Source: CAD feature listing. Evaluate the final solid. Frame: model axes, mm. A direction names the side the tool comes from. Give positions to 0.01 mm unless a question says otherwise; leave off trailing zeros. Order: outer loops, then holes, each group sorted by start corner. A loop starts at its lowest first (then second) coordinate and runs counter-clockwise, first axis right, second up. Notation, with made-up numbers: M 66,83 L 123,83 A27 ccw 123,122 Z; hole C 0,13.25 d3. An arc over 180 degrees is marked long. Use CSV: the item, a comma, the result in double quotes. Start each with the question number.
Item 1: Section query D-D on z = 16.5. Return loops of the section in (x, y), and give its area (3 significant figures).
Item 2: Section query B-B on z = 56. Return loops of the section in (x, y), and give its area (3 significant figures).
Item 3: Pull-direction query (Z, two-part tool) for faces 5 (the face through (3.1, 5.3, 45.72)), 6 (the face through (4.041, 3, 54)), 7 (the face through (0, 0, 0)), 8 (the face through (-1.26, -5.674, 26.146)); classes: +Z half, -Z half, draft (parallel to the pull), parting line (faces both ways), or undercut.
Item 4: Section query C-C on x = -5. Return loops of the section in (y, z).
Item 5: Access query for faces 1 (the face through (-3.639, 3, 54)), 2 (the face through (0, 5.812, 54)), 3 (the face through (-2.8, 5.4, 45.72)), 4 (the face through (0, 0.732, 54)). Directions: +Z, -Z, +X, -X, +Y, -Y. A direction counts if a zero-diameter tool reaches every point of the face in a straight line with its end or side. Return the directions, or none.
Item 6: First-contact query: pin 1 (10 mm diameter, centred on y = 7.5, z = 24.5, fed in from +X); pin 2 (8 mm diameter, centred on x = -8.5, z = 40.5, fed in from -Y); pin 3 (8.5 mm diameter, centred on x = -1, z = 57, fed in from +Y). Flat tips, straight axial feed; report the tip coordinate or a pass-through.
Item 7: Ray query, probe 1 along Z at (x, y) = (-2.5, 5.75); probe 2 along Z at (x, y) = (7.25, 2.25); probe 3 along X at (y, z) = (1.5, 51.5). Return the intervals inside material, ascending. Write a range as from..to.
Item 8: Section query A-A on y = 0. Return loops of the section in (x, z).
from build123d import *

# Parameters (mm, degrees)
F0_R     = 12.7
F1_DEPTH = 7.112
F2_R     = 5.811931
F3_DEPTH = 38.608
F5_DEPTH = 17.526


with BuildPart() as f1:
    # F0 (on Top) → F1 (new body)
    with BuildSketch(Plane.XY):
        Circle(F0_R)
    extrude(amount=F1_DEPTH)

    # F2 (on face) → F3 (join)
    with BuildSketch(Plane.XY.offset(7.112)):
        Circle(F2_R)
    extrude(amount=F3_DEPTH)

    # F4 (on face) → F5 (join)
    with BuildSketch(Plane.XY.offset(45.72)):
        with BuildLine():
            ThreePointArc((4.041356, 4.176839), (2.179798, 5.387673), (0, 5.811931))
            ThreePointArc((0, 5.811931), (-1.928979, 5.482479), (-3.639269, 4.531475))
            Line((-3.639269, 4.531475), (-3.639269, 0.731931))
            Line((-3.639269, 0.731931), (4.041356, 0.731931))
            Line((4.041356, 0.731931), (4.041356, 4.176839))
        make_face()
        with BuildLine():
            ThreePointArc((-3.639269, 4.531475), (-1.928979, 5.482479), (0, 5.811931))
            Line((0, 5.811931), (-3.639269, 5.811931))
            Line((-3.639269, 5.811931), (-3.639269, 4.531475))
        make_face()
        with BuildLine():
            Line((4.041356, 4.176839), (4.041356, 5.811931))
            Line((4.041356, 5.811931), (0, 5.811931))
            ThreePointArc((0, 5.811931), (2.179798, 5.387673), (4.041356, 4.176839))
        make_face()
    extrude(amount=F5_DEPTH)


solid = f1.part
Verdict:
1,outline,"C 0,0 d11.62"
1,area,"106 mm2"
2,outline,"M -3.64,0.73 L 4.04,0.73 L 4.04,5.81 L -3.64,5.81 Z"
2,area,"39.0 mm2"
3,face 5,"undercut"
3,face 6,"draft"
3,face 7,"-Z half"
3,face 8,"undercut"
4,outline,"M -11.67,0 L 11.67,0 L 11.67,7.11 L 2.96,7.11 L 2.96,45.72 L -2.96,45.72 L -2.96,7.11 L -11.67,7.11 Z"
5,face 1,"+Z, -X, +Y, -Y"
5,face 2,"+Z, +X, -X, +Y"
5,face 3,"-X, +Y"
5,face 4,"+Z, +X, -X, -Y"
6,pin 1,"x = 5.25"
6,pin 2,"y = -3.68"
6,pin 3,"y = 5.81"
7,probe 1,"0..7.11, 45.72..63.25"
7,probe 2,"0..7.11"
7,probe 3,"-3.64..4.04"
8,outline,"M -12.7,0 L 12.7,0 L 12.7,7.11 L 5.81,7.11 L 5.81,45.72 L -5.81,45.72 L -5.81,7.11 L -12.7,7.11 Z"
